Design review of the part built by this model. Coordinates are the model's own, in mm. Face numbers are marked on the shaded views. A direction names the side the tool comes from. Coordinates: 2 decimals unless noted, no trailing zeros. Order: outer loops, then holes, each group sorted by start corner. A loop starts at its lowest first (then second) coordinate and runs counter-clockwise, first axis right, second up. Notation, with made-up numbers: (29, 66) -> (50, 66) arc R13 cw to (50, 86) -> close; hole circle Ø4 at (35, -11). An arc over 180 degrees is marked (long way). Use a Markdown table: item, result. Add a question column.
Q1. Wall thickness on probe 1 along Z at (x, y) = (1.25, -0.5); probe 2 along X at (y, z) = (1.25, -2); probe 3 along Y at (x, z) = (-3, -2.25): over which ranges is each line inside the solid? List them lowest first.
Q2. Add section A-A (z = -3.75). State the section outline as (x, y) points, then the cut area to 3 significant figures.
Q3. Add section C-C (y = 0.5). State the section outline as (x, z) points.
Q4. Insertion check: pin 1 (1.5 mm diameter, centred on x = -2.5, z = -2, fed in from +Y); pin 2 (0.8 mm diameter, centred on y = -0.5, z = -2.5, fed in from -X); pin 3 (2 mm diameter, centred on y = -0.5, z = -2.5, fed in from +X). Each pin has a flat end and moves straight along its axis. Give the tip position at first contact, or say it passes through.
Q5. Machinability: for the marked faces 1, 2 and 3, which of the approach directions +Z, -Z, +X, -X, +Y, -Y give a long, thin tool a straight path to every point of the face, cutting with its end or side? Answer none if there is none.
Q6. Add section B-B (x = 1.25). State the section outline as (y, z) points, then the cut area to 3 significant figures.
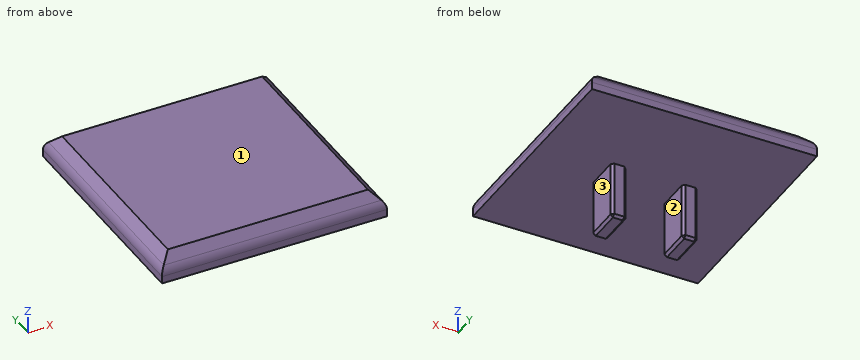
from build123d import *

# Parameters (mm, degrees)
SKETCH_W        = 18
SKETCH_H        = 18
PAD_DEPTH       = 2
CHAMFER_SIZE    = 1
FILLET_R        = 1
COPYSKETCH002_W = 1.2
COPYSKETCH002_H = 3
PAD001_DEPTH    = 4.5
CHAMFER001_SIZE = 0.2


with BuildPart() as part:
    # Sketch → Pad (new body)
    with BuildSketch(Plane.XY):
        Rectangle(SKETCH_W, SKETCH_H)
    extrude(amount=PAD_DEPTH)

    # Chamfer
    chamfer_edges = [part.edges().sort_by_distance(p)[0] for p in [
        (-9, 0, 2),
        (0, 9, 2),
        (9, 0, 2),
        (0, -9, 2),
    ]]
    chamfer(chamfer_edges, length=CHAMFER_SIZE)

    # Fillet
    fillet_edges = [part.edges().sort_by_distance(p)[0] for p in [
        (0, -9, 1),
        (9, 0, 1),
        (-9, 0, 1),
        (0, 9, 1),
    ]]
    fillet(fillet_edges, radius=FILLET_R)

    # CopySketch002 → Pad001 (join)
    with BuildSketch(Plane(origin=(0, 0, 0), x_dir=(1, 0, 0), z_dir=(0, 0, -1))):
        with Locations((-2.85, 0)):
            Rectangle(COPYSKETCH002_W, COPYSKETCH002_H)
        with Locations((2.85, 0)):
            Rectangle(COPYSKETCH002_W, COPYSKETCH002_H)
    extrude(amount=PAD001_DEPTH)

    # Chamfer001
    chamfer001_edges = [part.edges().sort_by_distance(p)[0] for p in [
        (-2.85, 1.5, -4.5),
        (-3.45, 0, -4.5),
        (-2.85, -1.5, -4.5),
        (-2.25, 0, -4.5),
        (-3.45, 1.5, -2.25),
        (-2.25, 1.5, -2.25),
        (-3.45, -1.5, -2.25),
        (-2.25, -1.5, -2.25),
        (2.85, -1.5, -4.5),
        (2.25, 0, -4.5),
        (2.85, 1.5, -4.5),
        (3.45, 0, -4.5),
        (3.45, -1.5, -2.25),
        (2.25, -1.5, -2.25),
        (2.25, 1.5, -2.25),
        (3.45, 1.5, -2.25),
    ]]
    chamfer(chamfer001_edges, length=CHAMFER001_SIZE)


solid = part.part
Established:
| question | item | result |
|---|---|---|
| 1 | probe 1 | 0 to 2 |
| 1 | probe 2 | -3.45 to -2.25, 2.25 to 3.45 |
| 1 | probe 3 | -1.5 to 1.5 |
| 2 | outline | (-3.45, -1.3) -> (-3.25, -1.5) -> (-2.45, -1.5) -> (-2.25, -1.3) -> (-2.25, 1.3) -> (-2.45, 1.5) -> (-3.25, 1.5) -> (-3.45, 1.3) -> close; (2.25, -1.3) -> (2.45, -1.5) -> (3.25, -1.5) -> (3.45, -1.3) -> (3.45, 1.3) -> (3.25, 1.5) -> (2.45, 1.5) -> (2.25, 1.3) -> close |
| 2 | area | 7.04 mm^2 |
| 3 | outline | (-9, 0) -> (-3.45, 0) -> (-3.45, -4.3) -> (-3.25, -4.5) -> (-2.45, -4.5) -> (-2.25, -4.3) -> (-2.25, 0) -> (2.25, 0) -> (2.25, -4.3) -> (2.45, -4.5) -> (3.25, -4.5) -> (3.45, -4.3) -> (3.45, 0) -> (9, 0) -> (9, 0.59) arc R1 ccw to (8.71, 1.29) -> (8, 2) -> (-8, 2) -> (-8.71, 1.29) arc R1 ccw to (-9, 0.59) -> close |
| 4 | pin 1 | y = 1.5 |
| 4 | pin 2 | x = -3.45 |
| 4 | pin 3 | x = 3.45 |
| 5 | face 1 | +Z, +X, -X, +Y, -Y |
| 5 | face 2 | -Z, +Y, -Y |
| 5 | face 3 | -Z, +X, +Y, -Y |
| 6 | outline | (-9, 0) -> (9, 0) -> (9, 0.59) arc R1 ccw to (8.71, 1.29) -> (8, 2) -> (-8, 2) -> (-8.71, 1.29) arc R1 ccw to (-9, 0.59) -> close |
| 6 | area | 35.0 mm^2 |
